Part model, mm, in its own coordinate system. A direction names the side the tool comes from. Coordinates: 2 decimals unless noted, no trailing zeros. Write each loop counter-clockwise with the first axis right and the second up, starting at its lowest first coordinate (ties: lowest second). Pieces come first, ordered by that corner, then holes. Notation, with made-up numbers: M 35,69 L 41,69 A29 ccw 41,93 Z; hole C -39.75,-39 d1. An arc over 180 degrees is marked long. Use a Markdown table: item, result. Add a question column.
Q1. Slice it at B-B on z = 6. Write the cut outline in (x, y).
Q2. Slice it at C-C on y = 10. Write the cut outline in (x, z), then the cut area to 3 significant figures.
Q3. Pin check, flat tips, straight feed: pin 1 Ø12 at (x, y) = (-18, 13.5) entering from -Z; pin 2 Ø12 at (x, z) = (-9.5, 17) entering from -Y. Stop position of each tip, or through.
Q4. Tool access for faces 4 (the cylindrical face through (14.9, 48.77, 5.93)), 5 (the flat face through (22.5, 13, 9)), 6 (the cylindrical face through (23.8, 8.2, 14.4)): list every direction of +Z, -Z, +X, -X, +Y, -Y with a clear straight run to the whole face (end or side of a thin tool).
Q5. Mould opens along Z. For faces 1 (the flat face through (25, 14, 12)), 2 (the flat face through (0, 49, 0)), 3 (the cylindrical face through (15.32, 48.77, 16.92)) say: released by +Z, released by -Z, zero draft, split by the parting line, or undercut.
Q6. Slice it at D-D on z = 12. Write the cut outline in (x, y), then the cut area to 4 significant figures.
Q7. Slice it at A-A on y = -0.5. Write the cut outline in (x, z), then the cut area to 3 significant figures.
Q8. Wall check: L1, parallel to X at y = 49.55, z = 18; L2, parallel to Z at x = 16.5, y = 48.2; L3, parallel to Y at x = 23.8, z = 12. Give the ranges that are in metal, low to high. Write a range as from..to.
from build123d import *

# Parameters (mm, degrees)
SKETCH_1_W                      = 50
SKETCH_1_H                      = 100
SKETCH_1_W_2                    = 45
SKETCH_1_H_2                    = 95
EXTRUDE_1_DEPTH                 = 24
SKETCH_3_R                      = 1.6
CUT_EXTRUDE_2_DEPTH             = 1
CUT_EXTRUDE_2_DEPTH_BACK        = 101
CUT_EXTRUDE_3_REACH             = 52
SKETCH_4_R                      = 3
SKETCH_4_R_2                    = 4
CUT_EXTRUDE_3_DIRECTION_2_DEPTH = 1
SKETCH_5_W                      = 50
SKETCH_5_H                      = 24
CUT_EXTRUDE_4_DEPTH             = 29


with BuildPart() as part:
    # ｽｹｯﾁ1 → ﾎﾞｽ - 押し出し1 (new body)
    with BuildSketch(Plane.XY):
        Rectangle(SKETCH_1_W, SKETCH_1_H)
        Rectangle(SKETCH_1_W_2, SKETCH_1_H_2, mode=Mode.SUBTRACT)
    extrude(amount=EXTRUDE_1_DEPTH)

    # ｽｹｯﾁ3 → ｶｯﾄ - 押し出し2 (cut, two sides)
    with BuildSketch(Plane(origin=(0, 50, 0), x_dir=(1, 0, 0), z_dir=(0, 1, 0))) as cut_extrude_2_sk:
        with Locations((-16.5, -6)):
            Circle(SKETCH_3_R)
        with Locations((16.5, -6)):
            Circle(SKETCH_3_R)
        with Locations((16.5, -18)):
            Circle(SKETCH_3_R)
        with Locations((-16.5, -18)):
            Circle(SKETCH_3_R)
    extrude(amount=CUT_EXTRUDE_2_DEPTH, mode=Mode.SUBTRACT)
    extrude(cut_extrude_2_sk.sketch, amount=-CUT_EXTRUDE_2_DEPTH_BACK, mode=Mode.SUBTRACT)

    # ｽｹｯﾁ4 → ｶｯﾄ - 押し出し3 (cut, up to next)
    with BuildSketch(Plane(origin=(25, 0, 0), x_dir=(0, 0, -1), z_dir=(1, 0, 0)), mode=Mode.PRIVATE) as cut_extrude_3_sk1:
        with Locations((-12, 10)):
            Circle(SKETCH_4_R)
    cut_extrude_3_tool1 = extrude(cut_extrude_3_sk1.sketch, amount=-CUT_EXTRUDE_3_REACH, mode=Mode.PRIVATE) & part.part
    add(cut_extrude_3_tool1.solids().sort_by_distance((25, 10, 12))[0], mode=Mode.SUBTRACT)
    # ｽｹｯﾁ4 → ｶｯﾄ - 押し出し3 (cut, up to next)
    with BuildSketch(Plane(origin=(25, 0, 0), x_dir=(0, 0, -1), z_dir=(1, 0, 0)), mode=Mode.PRIVATE) as cut_extrude_3_sk2:
        with Locations((-12, -30)):
            Circle(SKETCH_4_R_2)
    cut_extrude_3_tool2 = extrude(cut_extrude_3_sk2.sketch, amount=-CUT_EXTRUDE_3_REACH, mode=Mode.PRIVATE) & part.part
    add(cut_extrude_3_tool2.solids().sort_by_distance((25, -30, 12))[0], mode=Mode.SUBTRACT)

    # ｽｹｯﾁ4 → ｶｯﾄ - 押し出し3 direction 2 (cut)
    with BuildSketch(Plane(origin=(25, 0, 0), x_dir=(0, 0, -1), z_dir=(1, 0, 0))):
        with Locations((-12, 10)):
            Circle(SKETCH_4_R)
        with Locations((-12, -30)):
            Circle(SKETCH_4_R_2)
    extrude(amount=CUT_EXTRUDE_3_DIRECTION_2_DEPTH, mode=Mode.SUBTRACT)

    # ｽｹｯﾁ5 → ｶｯﾄ - 押し出し4 (cut)
    with BuildSketch(Plane.XZ.offset(50)):
        with Locations((0, 12)):
            Rectangle(SKETCH_5_W, SKETCH_5_H)
    extrude(amount=-CUT_EXTRUDE_4_DEPTH, mode=Mode.SUBTRACT)


solid = part.part
Recorded:
| question | item | result |
|---|---|---|
| 1 | outline | M -25,-21 L -22.5,-21 L -22.5,47.5 L -18.1,47.5 L -18.1,50 L -25,50 Z; M -14.9,47.5 L 14.9,47.5 L 14.9,50 L -14.9,50 Z; M 18.1,47.5 L 22.5,47.5 L 22.5,-21 L 25,-21 L 25,50 L 18.1,50 Z |
| 2 | outline | M -25,0 L -22.5,0 L -22.5,24 L -25,24 Z; M 22.5,0 L 25,0 L 25,9 L 22.5,9 Z; M 22.5,15 L 25,15 L 25,24 L 22.5,24 Z |
| 2 | area | 105 mm² |
| 3 | pin 1 | z = 0 |
| 3 | pin 2 | y = 47.5 |
| 4 | face 4 | +Y, -Y |
| 4 | face 5 | +Z, -Z, -Y |
| 4 | face 6 | +X |
| 5 | face 1 | zero draft |
| 5 | face 2 | released by -Z |
| 5 | face 3 | undercut |
| 6 | outline | M -25,-21 L -22.5,-21 L -22.5,47.5 L 22.5,47.5 L 22.5,13 L 25,13 L 25,50 L -25,50 Z; M 22.5,-21 L 25,-21 L 25,7 L 22.5,7 Z |
| 6 | area | 452.5 mm² |
| 7 | outline | M -25,0 L -22.5,0 L -22.5,24 L -25,24 Z; M 22.5,0 L 25,0 L 25,24 L 22.5,24 Z |
| 7 | area | 120 mm² |
| 8 | L1 | -25..-18.1, -14.9..14.9, 18.1..25 |
| 8 | L2 | 0..4.4, 7.6..16.4, 19.6..24 |
| 8 | L3 | -21..7, 13..50 |
